Check sheet for the modelled part. Datum: model origin and axes. Units: mm. Face numbers are marked on the shaded views. Give positions to 0.01 mm unless a question says otherwise; leave off trailing zeros. Loops run counter-clockwise (first coordinate to the right, second up) from the corner with the lowest first, then second, coordinate; pieces in that order, holes last.
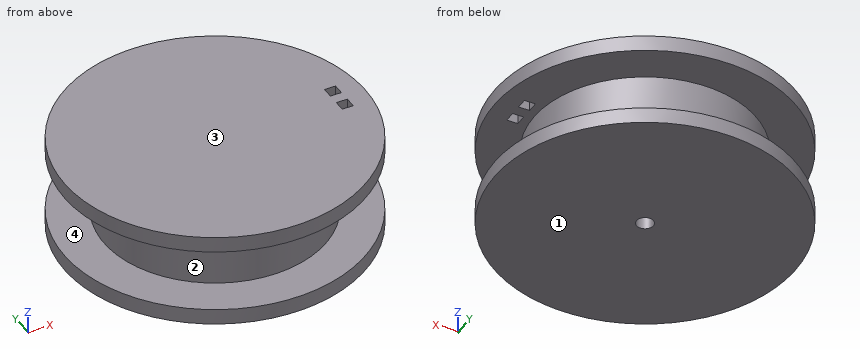
Autodesk Inventor part; units mm, degrees
ref_plane "YZ Plane" through (0, 0, 0) normal (1, 0, 0) x (0, 1, 0)
ref_plane "XZ Plane" through (0, 0, 0) normal (0, 1, 0) x (-1, 0, 0)
ref_plane "XY Plane" through (0, 0, 0) normal (0, 0, 1) x (1, 0, 0)
sketch "Sketch1" plane through (0, 0, 0) normal (0, 0, 1) x (1, 0, 0)
  circle A0 centre (0, 0) radius 35
  dimension "d0" = 70
extrude "Extrusion1" add sketch "Sketch1" along normal blind 20
sketch "Sketch2" plane through (0, 0, 20) normal (0, 0, 1) x (1, 0, 0)
  circle A0 centre (0, 0) radius 47.5
  dimension "d3" = 95
extrude "Extrusion2" add sketch "Sketch2" along normal blind 5
sketch "Sketch3" plane through (0, 0, 0) normal (0, 0, -1) x (-1, 0, 0)
  circle A0 centre (0, 0) radius 47.5
  dimension "d6" = 95
extrude "Extrusion3" add sketch "Sketch3" along normal blind 5
sketch "Sketch4" plane through (0, 0, -5) normal (0, 0, -1) x (-1, 0, 0)
  circle A0 centre (0, 0) radius 2.65
  line L0 (-2.65, 0) -> (2.03, 0)
  line L1 (2.03, 0) -> (2.03, -1.7034)
  line L2 (2.03, 0) -> (2.03, 1.7034)
  dimension "d9" = 5.3
  dimension "d10" = 4.68
extrude "Extrusion4" cut sketch "Sketch4" against normal blind 21 contours L2 L0 A0 | A0 L0 L1
extrude "Extrusion5" cut sketch "Sketch4" against normal blind 4 contours A0 L1 L2
sketch "Sketch5" plane through (0, 0, 25) normal (0, 0, 1) x (1, 0, 0)
  line L0 (57.5, 1.75) -> (37.5, 1.75)
  line L1 (37.5, 1.75) -> (37.5, -1.75)
  line L2 (37.5, -1.75) -> (57.5, -1.75)
  line L3 (57.5, -1.75) -> (57.5, 1.75)
  circle A0 centre (0, 0) radius 47.5
  line L4 (57.5, 1.75) -> (37.5, -1.75) construction
  line L5 (37.5, 1.75) -> (57.5, -1.75) construction
  line L6 (41, 5.25) -> (37.5, 5.25)
  line L7 (37.5, 5.25) -> (37.5, -5.25)
  line L8 (37.5, -5.25) -> (41, -5.25)
  line L9 (41, -5.25) -> (41, 5.25)
  point P0 (47.5, 0)
  point P1 (37.5, 0)
  point P2 (41, -1.75)
  point P3 (41, 1.75)
  point P4 (47.4678, 1.75)
  point P5 (47.4678, -1.75)
  dimension "d15" = 20
  dimension "d16" = 3.5
  dimension "d21" = 3.5
  dimension "d22" = 3.5
  dimension "d23" = 3.5
  dimension "d24" = 0
extrude "Extrusion6" cut sketch "Sketch5" against normal blind 10 contours L3 L2 A0 L0 | L0 L7 L6 L9 | L9 L8 L7 L2
equation "\"d6\" = d3"
properties part number "spool"
(1) Section check A-A on x = 0. Record the boundary of the cut face in (y, z).
(2) Section check C-C on z = 12.5. Record the boundary of the cut face in (x, y), plus the area to 3 significant figures.
(3) Section check B-B on y = 0. Record the boundary of the cut face in (x, z), plus the area to 3 significant figures.
(4) Release check for a two-part mould opening along Z. For the marked faces 1, 2, 3 and 4 record: pulls with the +Z half, pulls with the -Z half, needs draft (parallel to the pull), parting line crosses it, or undercut.
(5) Section check D-D on y = 27. Record the boundary of the cut face in (x, z).
(6) Gauge pin test, flat ends, axial feed: pin 1 Ø3 at (x, z) = (39.5, 23.5) entering from +Y; pin 2 Ø12 at (x, z) = (-26, 5.5) entering from +Y; pin 3 Ø5 at (x, z) = (6, 18) entering from -Y. Record the tip position at first contact, or that the pin passes through.
(7) Material ranges on line 1 (Z direction, x = -31.5, y = -31.5); line 2 (Y direction, x = 0, z = 8.25); line 3 (Y direction, x = 38, z = 22.25), recorded low to high.
Computed values:
1. outline: (-47.5, -5) - (-2.65, -5) - (-2.65, 16) - (2.65, 16) - (2.65, -5) - (47.5, -5) - (47.5, 0) - (35, 0) - (35, 20) - (47.5, 20) - (47.5, 25) - (-47.5, 25) - (-47.5, 20) - (-35, 20) - (-35, 0) - (-47.5, 0) - close
2. outline: circle Ø70 at (0, 0); hole (-2.03, -1.7) arc R2.65 ccw (long way) to (-2.03, 1.7) - close
2. area: 3,830 mm2
3. outline: (-47.5, -5) - (-2.65, -5) - (-2.65, -1) - (-2.03, -1) - (-2.03, 16) - (2.65, 16) - (2.65, -5) - (47.5, -5) - (47.5, 0) - (35, 0) - (35, 20) - (47.5, 20) - (47.5, 25) - (-47.5, 25) - (-47.5, 20) - (-35, 20) - (-35, 0) - (-47.5, 0) - close
3. area: 2,250 mm2
4. face 1: pulls with the -Z half
4. face 2: undercut
4. face 3: pulls with the +Z half
4. face 4: undercut
5. outline: (-39.08, -5) - (39.08, -5) - (39.08, 0) - (22.27, 0) - (22.27, 20) - (39.08, 20) - (39.08, 25) - (-39.08, 25) - (-39.08, 20) - (-22.27, 20) - (-22.27, 0) - (-39.08, 0) - close
6. pin 1: stops at y = 28.5
6. pin 2: stops at y = 41.22
6. pin 3: stops at y = -47.29
7. line 1: z = -5 to 0, 20 to 25
7. line 2: y = -35 to -2.65, 2.65 to 35
7. line 3: y = -28.5 to -5.25, -1.75 to 1.75, 5.25 to 28.5
